Autodesk Inventor part; units mm, degrees
ref_plane "screw_XY" through (0, 0, 0) normal (0, 1, 0) x (1, 0, 0)
ref_plane "screw_YZ" through (0, 0, 0) normal (1, 0, 0) x (0, 0, -1)
ref_plane "screw_ZX" through (0, 0, 0) normal (0, 0, -1) x (0, 1, 0)
sketch "Sketch_1" plane through (0, 0, 0) normal (0, 0, 1) x (1, 0, 0)
  line L0 (0, -1.1296) -> (0, 5.2204)
  line L1 (0, 5.2204) -> (1.6104, 5.2204)
  line L2 (1.6104, 5.2204) -> (2.0828, 4.748)
  line L3 (2.0828, 4.748) -> (2.0828, 0.1385)
  line L4 (2.0828, 0.1385) -> (3.4503, -1.009)
  line L5 (3.4503, -1.009) -> (3.4503, -1.1296)
  line L6 (3.4503, -1.1296) -> (0, -1.1296)
  line L7 (0, -1.1296) -> (0, 5.2204)
revolve "Revolution1" add sketch "Sketch_1" angle 360 about axis through (0, -1.1296, 0) along (0, -1, 0)
thread "Thread1"
sketch "Sketch_2" plane through (0, -1.1296, 0) normal (0, -1, 0) x (1, 0, 0)
  line L0 (-1.1906, -0.6874) -> (0, -1.3748)
  line L1 (0, -1.3748) -> (1.1906, -0.6874)
  line L2 (1.1906, -0.6874) -> (1.1906, 0.6874)
  line L3 (1.1906, 0.6874) -> (0, 1.3748)
  line L4 (0, 1.3748) -> (-1.1906, 0.6874)
  line L5 (-1.1906, 0.6874) -> (-1.1906, -0.6874)
extrude "Extrusion1" cut sketch "Sketch_2" against normal blind 0.7925
sketch "Sketch_3" plane through (0, 0, 0) normal (0, 0, 1) x (1, 0, 0)
  line L0 (0, -0.3371) -> (0, 0.3503)
  line L1 (0, 0.3503) -> (1.1906, -0.3371)
  line L2 (1.1906, -0.3371) -> (0, -0.3371)
  line L3 (0, -0.3371) -> (0, 0.3503)
revolve "Revolution2" cut sketch "Sketch_3" angle 360 about axis through (0, -0.3371, 0) along (0, -1, 0)
ref_plane "screw_XY" through (0, 0, 0) normal (0, 1, 0) x (1, 0, 0)
ref_plane "screw_YZ" through (0, 0, 0) normal (1, 0, 0) x (0, 0, -1)
ref_plane "screw_ZX" through (0, 0, 0) normal (0, 0, -1) x (0, 1, 0)
properties part number "8-32_1"
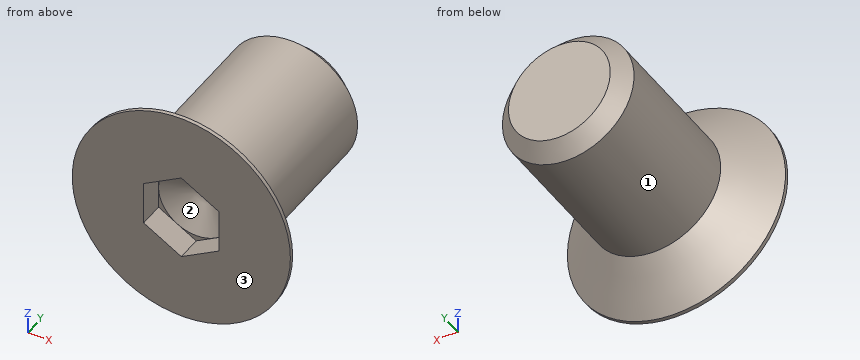
Geometry: final body of the model. Coordinates: model frame, mm. Face numbers are marked on the shaded views. Give positions to 0.01 mm unless a question says otherwise; leave off trailing zeros. Loops run counter-clockwise (first coordinate to the right, second up) from the corner with the lowest first, then second, coordinate; pieces in that order, holes last. Notation, with made-up numbers: M 63.5,62.25 L 104.5,62.25 A30 ccw 104.5,95.25 Z; hole C -23,59.5 d2. An arc over 180 degrees is marked long. Put each result on its own line as item: value. Start each with the question number.
1) Ray query, line 1 along Z through (x, y) = (-0.25, 0); line 2 along X through (y, z) = (-0.25, -0.5); line 3 along Z through (x, y) = (0, 0.5). Return the intervals inside material, ascending.
2) Cut plane B-B (y = 0). Output: boundary loops of the cut face in (x, z), then the cut area to 3 significant figures.
3) Pull-direction query (Z, two-part tool) for the marked faces 1, 2 and 3; classes: pulls with the +Z half, pulls with the -Z half, needs draft (parallel to the pull), parting line crosses it, or undercut.
4) Contact query for flat-ended pins moving along their axis: pin 1 (0.7 mm diameter, centred on x = -1, z = -0.5, fed in from -Y); pin 2 (1.5 mm diameter, centred on x = 2.5, y = 4.5, fed in from +Z); pin 3 (1.5 mm diameter, centred on x = 1.5, y = 2, fed in from +Z); pin 4 (3 mm diameter, centred on x = -0.5, y = 1, fed in from -Z). Output: stop coordinate, or through.
5) Cut plane A-A (y = 3). Output: boundary loops of the cut face in (x, z), then the cut area to 3 significant figures.
Verdict:
1. line 1: -2.23 to -0.55, 0.55 to 2.23
1. line 2: -2.5 to -0.91, 0.91 to 2.5
1. line 3: -2.08 to 2.08
2. outline: C 0,0 d4.5; hole C 0,0 d1.21
2. area: 14.7 mm2
3. face 1: parting line crosses it
3. face 2: undercut
3. face 3: needs draft
4. pin 1: y = -1.13
4. pin 2: z = 1.13
4. pin 3: z = 1.94
4. pin 4: z = -2.81
5. outline: C 0,0 d4.17
5. area: 13.6 mm2
